Work out the finished part from the listing and answer in its coordinate system (mm). A direction names the side the tool comes from. Round coordinates to 2 decimals unless told otherwise and drop trailing zeros. Loops run counter-clockwise (first coordinate to the right, second up) from the corner with the lowest first, then second, coordinate; pieces in that order, holes last.
Autodesk Inventor part; units mm, degrees
ref_plane "YZ Plane" through (0, 0, 0) normal (1, 0, 0) x (0, 1, 0)
ref_plane "XZ Plane" through (0, 0, 0) normal (0, 1, 0) x (-1, 0, 0)
ref_plane "XY Plane" through (0, 0, 0) normal (0, 0, 1) x (1, 0, 0)
sketch "Sketch1" plane through (0, 0, 0) normal (0, 0, 1) x (1, 0, 0)
  line L0 (0, 0) -> (25.4, 0)
  line L1 (25.4, 0) -> (25.4, 25.4)
  line L2 (25.4, 25.4) -> (0, 25.4)
  line L3 (0, 25.4) -> (0, 0)
  line L4 (1.5875, 23.8125) -> (23.8125, 23.8125)
  line L5 (23.8125, 23.8125) -> (23.8125, 1.5875)
  line L6 (23.8125, 1.5875) -> (1.5875, 1.5875)
  line L7 (1.5875, 1.5875) -> (1.5875, 23.8125)
  dimension "d0" = 25.4
  dimension "d1" = 25.4
  dimension "d4" = 1.5875
extrude "Extrusion1" add sketch "Sketch1" against normal blind 25.4 contours L3 L2 L1 L0 | L4 L5 L6 L7
extrude "Extrusion2" add sketch "Sketch1" along normal blind 25.4 contours L4 L5 L6 L7
sketch "Sketch2" plane through (25.4, 0, 0) normal (1, 0, 0) x (0, 0, -1)
  line L0 (25.4, 0) -> (25.4, 25.4)
  line L1 (0, 25.4) -> (25.4, 25.4)
  line L2 (0, 0) -> (0, 25.4)
  line L3 (0, 0) -> (25.4, 0)
  line L4 (23.8125, 23.8125) -> (23.8125, 1.5875)
  line L5 (23.8125, 1.5875) -> (1.5875, 1.5875)
  line L6 (1.5875, 1.5875) -> (1.5875, 23.8125)
  line L7 (1.5875, 23.8125) -> (23.8125, 23.8125)
  dimension "d8" = 1.5875
sketch "Sketch3" plane through (0, 25.4, 0) normal (0, 1, 0) x (1, 0, 0)
  line L0 (25.4, 25.4) -> (0, 25.4)
  line L1 (0, 0) -> (0, 25.4)
  line L2 (25.4, 0) -> (0, 0)
  line L3 (25.4, 0) -> (25.4, 25.4)
  line L4 (1.5875, 23.8125) -> (23.8125, 23.8125)
  line L5 (23.8125, 23.8125) -> (23.8125, 1.5875)
  line L6 (23.8125, 1.5875) -> (1.5875, 1.5875)
  line L7 (1.5875, 1.5875) -> (1.5875, 23.8125)
  dimension "d9" = 1.5875
extrude "Extrusion3" add sketch "Sketch2" along normal blind 25.4 contours L4 L5 L6 L7
extrude "Extrusion4" add sketch "Sketch3" along normal blind 25.4 contours L4 L5 L6 L7
sketch "Sketch4" plane through (0, 0, 0) normal (-1, 0, 0) x (0, 0, 1)
  line L0 (-25.4, 25.4) -> (-25.4, 0)
  line L1 (0, 0) -> (-25.4, 0)
  line L2 (0, 25.4) -> (0, 0)
  line L3 (0, 25.4) -> (-25.4, 25.4)
  line L4 (-23.8125, 23.8125) -> (-23.8125, 1.5875)
  line L5 (-23.8125, 1.5875) -> (-1.5875, 1.5875)
  line L6 (-1.5875, 1.5875) -> (-1.5875, 23.8125)
  line L7 (-1.5875, 23.8125) -> (-23.8125, 23.8125)
  dimension "d15" = 1.5875
extrude "Extrusion5" add sketch "Sketch4" along normal blind 25.4 contours L7 L6 L5 L4
sketch "Sketch5" plane through (0, 0, -25.4) normal (0, 0, -1) x (-1, 0, 0)
  line L0 (-25.4, 0) -> (-25.4, 25.4)
  line L1 (0, 0) -> (-25.4, 0)
  line L2 (0, 25.4) -> (0, 0)
  line L3 (-25.4, 25.4) -> (0, 25.4)
  line L4 (-1.5875, 23.8125) -> (-1.5875, 1.5875)
  line L5 (-1.5875, 1.5875) -> (-23.8125, 1.5875)
  line L6 (-23.8125, 1.5875) -> (-23.8125, 23.8125)
  line L7 (-23.8125, 23.8125) -> (-1.5875, 23.8125)
  dimension "d18" = 1.5875
extrude "Extrusion6" add sketch "Sketch5" along normal blind 25.4 contours L4 L5 L6 L7
sketch "Sketch7" plane through (1.5875, 23.8125, -25.4) normal (0, 1, 0) x (1, 0, 0)
  line L0 (22.225, 0) -> (0, 0)
  line L1 (23.8125, -25.4) -> (-1.5875, -25.4)
  line L2 (23.8125, -25.4) -> (23.8125, 0)
  point P0 (11.1125, -38.1)
  point P1 (-14.2875, -12.7)
  point P2 (11.1125, 12.7)
  point P3 (36.5125, -12.7)
  dimension "d26" = 12.7
  dimension "d28" = 12.7
  dimension "d29" = 12.7
  dimension "d52" = 12.7
  dimension "d53" = 50.8
hole "Hole1" at (12.7, 23.8125, 12.7) at (-12.7, 23.8125, -12.7) at (12.7, 23.8125, -38.1) at (38.1, 23.8125, -12.7) direction (0, -1, 0) diameter 6.35 depth 25.4 tip angle 118
sketch "Sketch8" plane through (1.5875, 25.4, -23.8125) normal (-1, 0, 0) x (0, 0, 1)
  point P0 (23.8125, -25.4)
  point P1 (11.1125, 12.7)
hole "Hole2" at (1.5875, 38.1, -12.7) direction (1, 0, 0) diameter 6.35 depth 25.4 tip angle 118
sketch "Sketch9" plane through (23.8125, 25.4, -23.8125) normal (0, 0, -1) x (-1, 0, 0)
  point P0 (23.8125, -25.4)
  point P1 (11.1125, 12.7)
hole "Hole3" at (12.7, 38.1, -23.8125) direction (0, 0, 1) diameter 6.35 depth 25.4 tip angle 118
properties part number "5-way corner"
Item 1: Section B-B, the plane x = 38.1 is taken. Give the vertices of the cut face in (y, z) (1 decimal).
Item 2: Straight lines are drawn through the part: line 1 (X direction, y = 14.75, z = -12.7) (3 decimals); line 2 (X direction, y = 38.1, z = -17) (1 decimal); line 3 (Z direction, x = 13.5, y = 14). For each, find the intervals that lie inside material, in ascending order.
Item 3: Section A-A, the plane z = -38.1 is taken. Give the vertices of the cut face in (x, y) (1 decimal).
Item 4: For faces 1 (the face through (1.588, 13, 13)), 2 (the face through (10, 35, -23.812)), 3 (the face through (15, 35, -1.588)), 4 (the face through (38, 13, -23.812)), determine the directions among +Z, -Z, +X, -X, +Y, -Y from which every point of the face is accessible in a straight line to the end or side of a thin tool.
Item 5: Each of these flat-tipped pins is pushed along its axis until it touches: P1, Ø18, axis at x = 41, z = -11, coming from the +Y side; P2, Ø24.5, axis at x = -14, y = 14, coming from the +Z side; P3, Ø11, axis at x = -16.5, z = -11.5, coming from the -Y side. Where does it stop, or does it pass through?
Item 6: Determine the mould class of faces 5 (the face through (13, 50.8, -13)), 6 (the face through (-15.3, 1.588, -15.3)), 7 (the face through (-9.9, 12.5, -11.2)) for opening direction Y: pulls with the +Y half, pulls with the -Y half, needs draft (parallel to the pull), parting line crosses it, or undercut.
Item 7: Section C-C, the plane y = 38.1 is taken. Give the vertices of the cut face in (x, z) (1 decimal).
Answer below:
1. outline: (1.6, -23.8) - (23.8, -23.8) - (23.8, -15.9) - (1.6, -15.9) - close; (1.6, -9.5) - (23.8, -9.5) - (23.8, -1.6) - (1.6, -1.6) - close
2. line 1: x = -25.4 to -15.875, -9.525 to 34.925, 41.275 to 50.8
2. line 2: x = 1.6 to 9.5, 15.9 to 23.8
2. line 3: z = -50.8 to -41.17, -35.03 to 9.63, 15.77 to 25.4
3. outline: (1.6, 1.6) - (9.5, 1.6) - (9.5, 23.8) - (1.6, 23.8) - close; (15.9, 1.6) - (23.8, 1.6) - (23.8, 23.8) - (15.9, 23.8) - close
4. face 1: +Z, -X, +Y, -Y
4. face 2: -Z, +X, -X, +Y
4. face 3: +Z, +X, -X, +Y
4. face 4: -Z, +X, +Y, -Y
5. P1: stops at y = 23.81
5. P2: stops at z = -1.59
5. P3: stops at y = 1.59
6. face 5: pulls with the +Y half
6. face 6: pulls with the -Y half
6. face 7: needs draft
7. outline: (1.6, -23.8) - (9.5, -23.8) - (9.5, -15.9) - (1.6, -15.9) - close; (1.6, -9.5) - (9.5, -9.5) - (9.5, -1.6) - (1.6, -1.6) - close; (15.9, -23.8) - (23.8, -23.8) - (23.8, -15.9) - (15.9, -15.9) - close; (15.9, -9.5) - (23.8, -9.5) - (23.8, -1.6) - (15.9, -1.6) - close
